The listing builds one solid part. Answer for the finished solid, in the listing's coordinates (mm). A direction names the side the tool comes from. Coordinates: 2 decimals unless noted, no trailing zeros. Loops run counter-clockwise (first coordinate to the right, second up) from the corner with the lowest first, then second, coordinate; pieces in that order, holes last. Notation, with made-up numbers: M 60.25,-12 L 107.25,-12 A21 ccw 107.25,1 Z; hole C 84.5,67 d1. An arc over 180 degrees is marked long. Return JSON: item names as keys, results as strings. Group by question number.
1. The mould has two halves that part along X. Classify faces 6 (the face through (-54, 8.137, 8)), 7 (the face through (22.181, 6, 7)), 8 (the face through (29.181, 17, 11)): pulls with the +X half, pulls with the -X half, needs draft (parallel to the pull), parting line crosses it, or undercut.
2. Given P1, Ø2, axis at x = -23, z = 7, coming from the +Y side; P2, Ø3, axis at y = 9.5, z = 6.5, coming from the +X side; P3, Ø1.5, axis at x = -35.5, y = 16.5, coming from the -Z side; P4, Ø3.5, axis at x = -125.32, y = -4.36, coming from the -Z side, each flat-ended and moving along its own axis, determine where each tip first touches the part or whether it passes through.
3. Section A-A (x = -13) is taken. Write down the section's boundary in (y, z), then the cut area to 3 significant figures.
4. Straight lines are drawn through the part: L1, parallel to X at y = -0.5, z = 8; L2, parallel to X at y = 1, z = 3.5; L3, parallel to Y at x = -97, z = 12. For each, find the intervals that lie inside material, in ascending order. Write a range as from..to.
5. Which of the six approach directions +Z, -Z, +X, -X, +Y, -Y give full straight-line access (tool end or side, diameter ignored) to faces 1 (the face through (-31, 23.137, 11)), 2 (the face through (-123.466, 4.686, 3.217)), 3 (the face through (-88.819, 21, 13)), 4 (the face through (-118, -4, 2.6)), 5 (the face through (-110, -4, 3))?
```python
from build123d import *
from OCP.BRepFilletAPI import BRepFilletAPI_MakeChamfer

# Parameters (mm, degrees)
BOSS_EXTRUDE1_DEPTH      = 14
BOSS_EXTRUDE1_DEPTH_BACK = 14
CUT_EXTRUDE1_DEPTH       = 157
CUT_EXTRUDE4_DEPTH       = 2.5
CUT_EXTRUDE4_DEPTH_BACK  = 2.5
SKETCH8_W                = 125
SKETCH8_H                = 34.7
CUT_EXTRUDE5_DEPTH       = 131.960317585
CUT_EXTRUDE5_DEPTH_BACK  = 131.960317585
SKETCH9_R                = 2.7
CHAMFER2_SIZE            = 5
CHAMFER2_SIZE_2          = 0.262038896
CUT_EXTRUDE8_DEPTH       = 7
CUT_EXTRUDE9_DEPTH       = 131.749429849
SKETCH16_W               = 214.344642296
SKETCH16_H               = 84.645654919
CUT_EXTRUDE10_DEPTH      = 131.960317585
SKETCH17_W               = 2
SKETCH17_H               = 14.7
CUT_EXTRUDE11_DEPTH      = 9.8
SKETCH18_R               = 1.35
CUT_EXTRUDE12_DEPTH      = 3
CHAMFER7_SIZE            = 3.5
SKETCH19_W               = 5
SKETCH19_H               = 7.5
BOSS_EXTRUDE2_DEPTH      = 2


with BuildPart() as part:
    # Sketch1 → Boss-Extrude1 (new, two sides: drawn at the far end of the back side and taken through both)
    with BuildSketch(Plane.XY.offset(-BOSS_EXTRUDE1_DEPTH_BACK)):
        Polygon((-127.819104229, -9.862903226), (22.180895771, -9.862903226), (22.180895771, -2.612903226), (27.180895771, -2.612903226), (27.180895771, 2.887096774), (22.180895771, 2.887096774), (22.180895771, 10.137096774), (31.180895771, 10.137096774), (31.180895771, 23.637096774), (31.180895771, 24.837096774), (-88.819104229, 24.837096774), (-88.819104229, 23.637096774), (-88.819104229, 15.637096774), (-127.819104229, 15.637096774), align=None)
    extrude(amount=BOSS_EXTRUDE1_DEPTH + BOSS_EXTRUDE1_DEPTH_BACK)

    # Sketch2 → Cut-Extrude1 (cut)
    with BuildSketch(Plane.ZY.offset(127.819104229)):
        Polygon((-12.8, 23.137096774), (-12.8, 8.137096774), (12.8, 8.137096774), (12.8, 23.137096774), (9.8, 23.137096774), (9.8, 24.837096774), (-9.8, 24.837096774), (-9.8, 23.137096774), align=None)
    extrude(amount=-CUT_EXTRUDE1_DEPTH, mode=Mode.SUBTRACT)

    # Sketch8 → Cut-Extrude4 (cut, two sides: drawn at the far end of the back side and taken through both)
    with BuildSketch(Plane.XY.offset(-CUT_EXTRUDE4_DEPTH_BACK)):
        with Locations((-45.319104229, 7.487096774)):
            Rectangle(SKETCH8_W, SKETCH8_H)
    extrude(amount=CUT_EXTRUDE4_DEPTH + CUT_EXTRUDE4_DEPTH_BACK, mode=Mode.SUBTRACT)

    # Sketch9 → Cut-Extrude5 (cut, two sides: drawn at the far end of the back side and taken through both)
    with BuildSketch(Plane.XY.offset(-CUT_EXTRUDE5_DEPTH_BACK)):
        with Locations((-77.819104229, -0.862903226)):
            Circle(SKETCH9_R)
        with Locations((2.180895771, -0.862903226)):
            Circle(SKETCH9_R)
    extrude(amount=CUT_EXTRUDE5_DEPTH + CUT_EXTRUDE5_DEPTH_BACK, mode=Mode.SUBTRACT)

    # Chamfer2
    chamfer2_edges_1 = [part.edges().sort_by_distance(p)[0] for p in [
        (27.180895771, -2.612903226, 0),
    ]]
    chamfer2_side_1 = [part.faces().sort_by_distance(p)[0] for p in [
        (27.175654993, -2.612903226, 0),
    ]]
    chamfer2_edges_2 = [part.edges().sort_by_distance(p)[0] for p in [
        (27.180895771, 2.887096774, 0),
    ]]
    chamfer2_side_2 = [part.faces().sort_by_distance(p)[0] for p in [
        (27.180895771, 2.881855996, 0),
    ]]
    chamfer2 = BRepFilletAPI_MakeChamfer(part.part.solid().wrapped)
    for e in chamfer2_edges_1:
        chamfer2.Add(CHAMFER2_SIZE - 0.0001, CHAMFER2_SIZE_2 - 0.0001, e.wrapped, chamfer2_side_1[0].wrapped)
    for e in chamfer2_edges_2:
        chamfer2.Add(CHAMFER2_SIZE_2 - 0.0001, CHAMFER2_SIZE - 0.0001, e.wrapped, chamfer2_side_2[0].wrapped)
    add(Compound.cast(chamfer2.Shape()), mode=Mode.REPLACE)  # a hair under: the kernel refuses the full size

    # Sketch14 → Cut-Extrude8 (cut)
    with BuildSketch(Plane(origin=(0, 8.137096774, 0), x_dir=(1, 0, 0), z_dir=(0, 1, 0))):
        with BuildLine():
            Line((-120.319104229, 4.5), (-115.319104229, 4.5))
            ThreePointArc((-115.319104229, 4.5), (-110.819104229, 0), (-115.319104229, -4.5))
            Line((-115.319104229, -4.5), (-120.319104229, -4.5))
            ThreePointArc((-120.319104229, -4.5), (-124.819104229, 0), (-120.319104229, 4.5))
        make_face()
    extrude(amount=-CUT_EXTRUDE8_DEPTH, mode=Mode.SUBTRACT)

    # Sketch15 → Cut-Extrude9 (cut, through all)
    with BuildSketch(Plane(origin=(0, 1.137096774, 0), x_dir=(1, 0, 0), z_dir=(0, 1, 0))):
        with BuildLine():
            Line((-120.319104229, -2.6), (-115.319104229, -2.6))
            ThreePointArc((-115.319104229, -2.6), (-112.719104229, 0), (-115.319104229, 2.6))
            Line((-115.319104229, 2.6), (-120.319104229, 2.6))
            ThreePointArc((-120.319104229, 2.6), (-122.919104229, 0), (-120.319104229, -2.6))
        make_face()
    extrude(amount=-CUT_EXTRUDE9_DEPTH, mode=Mode.SUBTRACT)

    # Sketch16 → Cut-Extrude10 (cut, through all)
    with BuildSketch(Plane.XY):
        with Locations((-30.272765953, 16.776086779)):
            Rectangle(SKETCH16_W, SKETCH16_H)
    extrude(amount=-CUT_EXTRUDE10_DEPTH, mode=Mode.SUBTRACT)

    # Sketch17 → Cut-Extrude11 (cut)
    with BuildSketch(Plane(origin=(0, 0, 0), x_dir=(-1, 0, 0), z_dir=(0, 0, -1))):
        with Locations((-30.180895771, 17.487096774)):
            Rectangle(SKETCH17_W, SKETCH17_H)
    extrude(amount=-CUT_EXTRUDE11_DEPTH, mode=Mode.SUBTRACT)

    # Sketch18 → Cut-Extrude12 (cut)
    with BuildSketch(Plane(origin=(0, 0, 0), x_dir=(-1, 0, 0), z_dir=(0, 0, -1))):
        with Locations((110.319104229, -4.362903226)):
            Circle(SKETCH18_R)
        with Locations((125.319104229, -4.362903226)):
            Circle(SKETCH18_R)
        with Locations((-22.180895771, 0.137096774)):
            Circle(SKETCH18_R)
    extrude(amount=-CUT_EXTRUDE12_DEPTH, mode=Mode.SUBTRACT)

    # Chamfer7
    chamfer7_edges = [part.edges().sort_by_distance(p)[0] for p in [
        (-80.519104229, -0.862903226, 14),
        (-0.519104229, -0.862903226, 14),
    ]]
    chamfer(chamfer7_edges, length=CHAMFER7_SIZE)

    # Sketch19 → Boss-Extrude2 (add)
    with BuildSketch(Plane(origin=(0, 0, 12.8), x_dir=(-1, 0, 0), z_dir=(0, 0, -1))):
        with Locations((93.819104229, 11.887096774)):
            Rectangle(SKETCH19_W, SKETCH19_H)
    extrude(amount=BOSS_EXTRUDE2_DEPTH)


solid = part.part
```
Worked out:
{
 "1": {"face 6": "needs draft", "face 7": "pulls with the +X half", "face 8": "undercut"},
 "2": {"P1": "y = 8.14", "P2": "x = 22.18", "P3": "z = 12.8", "P4": "z = 0"},
 "3": {"outline": "M -9.86,2.5 L 8.14,2.5 L 8.14,12.8 L 23.14,12.8 L 23.14,9.8 L 24.84,9.8 L 24.84,14 L -9.86,14 Z", "area": "232 mm^2"},
 "4": {"L1": "-127.82..-80.49, -75.14..-0.49, 4.86..27.18", "L2": "-127.82..-79.77, -75.86..0.23, 4.14..27.18", "L3": "-9.86..8.14"},
 "5": {"face 1": "-Z, -X", "face 2": "-Z, +Y", "face 3": "+Z, -Z, -X, +Y", "face 4": "-Z, +Y, -Y", "face 5": "-Z"}
}
